Model file for the job. Use its own axes, mm. Give positions to 0.01 mm unless a question says otherwise; leave off trailing zeros. Write each loop counter-clockwise with the first axis right and the second up, starting at its lowest first coordinate (ties: lowest second). Pieces come first, ordered by that corner, then holes. Notation, with made-up numbers: (67.25, 87) - (98.25, 87) arc R14 cw to (98.25, 92) - close; hole circle Ø3 at (-2, 21.5). An arc over 180 degrees is marked (long way). Use a Markdown table: item, result. Add a question column.
```python
from build123d import *

# Parameters (mm, degrees)
SKETCH_1_W      = 44
SKETCH_1_H      = 50
SKETCH_1_R      = 1.5
EXTRUDE_1_DEPTH = 3
FILLET_1_R      = 3
SKETCH_2_W      = 2.54
SKETCH_2_H      = 20.32
EXTRUDE_2_DEPTH = 0.5


with BuildPart() as part:
    # 草图1 → 凸台-拉伸1 (new body)
    with BuildSketch(Plane(origin=(0, 0, 0), x_dir=(1, 0, 0), z_dir=(0, 1, 0))):
        Rectangle(SKETCH_1_W, SKETCH_1_H)
        with Locations(Location((-10, 10, 0), (0, 0, 270))):
            Circle(SKETCH_1_R, mode=Mode.SUBTRACT)
        with Locations(Location((10, 10, 0), (0, 0, 90))):
            Circle(SKETCH_1_R, mode=Mode.SUBTRACT)
        with Locations(Location((10, -10, 0), (0, 0, 270))):
            Circle(SKETCH_1_R, mode=Mode.SUBTRACT)
        with Locations(Location((-10, -10, 0), (0, 0, 90))):
            Circle(SKETCH_1_R, mode=Mode.SUBTRACT)
        with Locations(Location((-14.75, 21, 0), (0, 0, 270))):
            Circle(SKETCH_1_R, mode=Mode.SUBTRACT)
        with Locations(Location((14.75, 21, 0), (0, 0, 90))):
            Circle(SKETCH_1_R, mode=Mode.SUBTRACT)
    extrude(amount=EXTRUDE_1_DEPTH)

    # 圆角1
    fillet_1_edges = [part.edges().sort_by_distance(p)[0] for p in [
        (22, 1.5, 25),
        (-22, 1.5, 25),
        (-22, 1.5, -25),
        (22, 1.5, -25),
    ]]
    fillet(fillet_1_edges, radius=FILLET_1_R)

    # 草图2 → 凸台-拉伸2 (add)
    with BuildSketch(Plane(origin=(0, 3, 0), x_dir=(1, 0, 0), z_dir=(0, 1, 0))):
        with Locations((-16.73, -11.84)):
            Rectangle(SKETCH_2_W, SKETCH_2_H)
        with Locations((16.73, -11.84)):
            Rectangle(SKETCH_2_W, SKETCH_2_H)
    extrude(amount=EXTRUDE_2_DEPTH)


solid = part.part
```
(1) Two-plate mould, pull along Z, no slides. Class faces 1 (the flat face through (22, 1, 0)), 2 (the flat face through (0, 1, -25)), 3 (the cylindrical face through (10.9, 1.5, -8.8)), 4 (the cylindrical face through (-9.1, 1.5, 11.2)): +Z half, -Z half, draft (parallel to the pull), parting line (faces both ways), or undercut.
(2) Band-saw the part on C-C (y = 1.55). Write the cut outline in (x, z), then the cut area to 3 significant figures.
(3) Band-saw the part on D-D (x = -10). Write the cut outline in (y, z).
(4) Band-saw the part on B-B (x = 14.75). Write the cut outline in (y, z), then the cut area to 3 significant figures.
(5) Flat gauge pins, fed straight in: pin 1 (4 mm diameter, centred on x = -6.5, z = -3.5, fed in from +Y); pin 2 (0.6 mm diameter, centred on y = 3.5, z = 13.5, fed in from -X); pin 3 (0.6 mm diameter, centred on x = 17, y = 3.5, fed in from +Z). Where does each tip first touch, or does it go through?
(6) Band-saw the part on A-A (z = 10). Write the cut outline in (x, y).
(7) Probe probe 1 along X at (y, z) = (2.2, 10); probe 2 along X at (y, z) = (2.3, -21); probe 3 along Z at (x, y) = (14.75, 0.95). List the from-to ranges inside material, lowest first. Write a range as [from, to].
Model answer:
| question | item | result |
|---|---|---|
| 1 | face 1 | draft |
| 1 | face 2 | -Z half |
| 1 | face 3 | undercut |
| 1 | face 4 | undercut |
| 2 | outline | (-22, -22) arc R3 ccw to (-19, -25) - (19, -25) arc R3 ccw to (22, -22) - (22, 22) arc R3 ccw to (19, 25) - (-19, 25) arc R3 ccw to (-22, 22) - close; hole circle Ø3 at (-14.75, -21); hole circle Ø3 at (-10, -10); hole circle Ø3 at (-10, 10); hole circle Ø3 at (10, -10); hole circle Ø3 at (10, 10); hole circle Ø3 at (14.75, -21) |
| 2 | area | 2,150 mm^2 |
| 3 | outline | (0, -25) - (3, -25) - (3, -11.5) - (0, -11.5) - close; (0, -8.5) - (3, -8.5) - (3, 8.5) - (0, 8.5) - close; (0, 11.5) - (3, 11.5) - (3, 25) - (0, 25) - close |
| 4 | outline | (0, -25) - (3, -25) - (3, -22.5) - (0, -22.5) - close; (0, -19.5) - (3, -19.5) - (3, 25) - (0, 25) - close |
| 4 | area | 141 mm^2 |
| 5 | pin 1 | stops at y = 3 |
| 5 | pin 2 | stops at x = -18 |
| 5 | pin 3 | stops at z = 22 |
| 6 | outline | (-22, 0) - (-11.5, 0) - (-11.5, 3) - (-15.46, 3) - (-15.46, 3.5) - (-18, 3.5) - (-18, 3) - (-22, 3) - close; (-8.5, 0) - (8.5, 0) - (8.5, 3) - (-8.5, 3) - close; (11.5, 0) - (22, 0) - (22, 3) - (18, 3) - (18, 3.5) - (15.46, 3.5) - (15.46, 3) - (11.5, 3) - close |
| 7 | probe 1 | x = [-22, -11.5], [-8.5, 8.5], [11.5, 22] |
| 7 | probe 2 | x = [-22, -16.25], [-13.25, 13.25], [16.25, 22] |
| 7 | probe 3 | z = [-25, -22.5], [-19.5, 25] |
